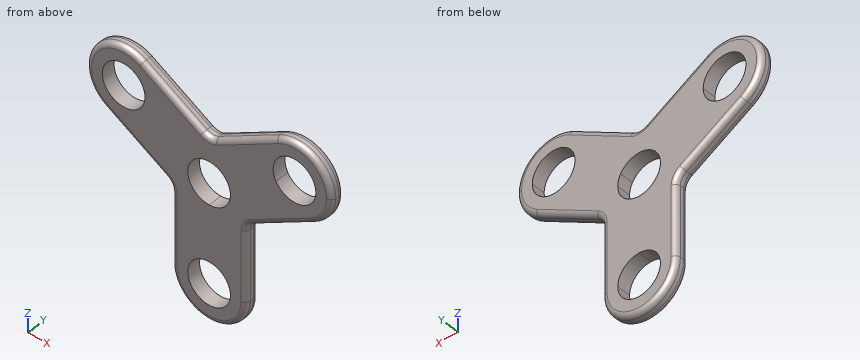
from build123d import *

# Parameters (mm, degrees)
F1_DEPTH = 6.9977
F2_R     = 2.54


with BuildPart() as f1:
    # F0 (on Front) → F1 (new body)
    with BuildSketch(Plane.XZ):
        with BuildLine():
            ThreePointArc((16.4977839421, 15.875), (18.4008869908, 11.2805028092), (19.05, 6.35))
            ThreePointArc((19.05, 6.35), (13.4703841816, -7.1203841816), (0, -12.7))
            Line((0, -12.7), (0, -25.4))
            ThreePointArc((0, -25.4), (13.4703841816, -30.9796158184), (19.05, -44.45))
            Line((19.05, -44.45), (19.05, -8.3146968374))
            ThreePointArc((19.05, -8.3146968374), (19.900738686, -5.1396968374), (22.225, -2.8154355234))
            Line((22.225, -2.8154355234), (53.5190905122, 15.2522160579))
            ThreePointArc((53.5190905122, 15.2522160579), (39.063587703, 13.3491130092), (27.4963065702, 22.225))
            Line((27.4963065702, 22.225), (16.4977839421, 15.875))
        make_face()
        with BuildLine():
            ThreePointArc((-16.4977839421, 15.875), (0, 25.4), (16.4977839421, 15.875))
            Line((16.4977839421, 15.875), (27.4963065702, 22.225))
            ThreePointArc((27.4963065702, 22.225), (25.5932035214, 36.6805028092), (34.4690905122, 48.2477839421))
            Line((34.4690905122, 48.2477839421), (3.175, 30.1801323608))
            ThreePointArc((3.175, 30.1801323608), (0, 29.3293936748), (-3.175, 30.1801323608))
            Line((-3.175, 30.1801323608), (-34.4690905122, 48.2477839421))
            ThreePointArc((-34.4690905122, 48.2477839421), (-27.4963065702, 41.275), (-24.9440905122, 31.75))
            ThreePointArc((-24.9440905122, 31.75), (-25.5932035214, 26.8194971908), (-27.4963065702, 22.225))
            Line((-27.4963065702, 22.225), (-16.4977839421, 15.875))
        make_face()
        with BuildLine():
            Line((0, -25.4), (0, -12.7))
            ThreePointArc((0, -12.7), (-16.4977839421, -3.175), (-16.4977839421, 15.875))
            Line((-16.4977839421, 15.875), (-27.4963065702, 22.225))
            ThreePointArc((-27.4963065702, 22.225), (-39.063587703, 13.3491130092), (-53.5190905122, 15.2522160579))
            Line((-53.5190905122, 15.2522160579), (-22.225, -2.8154355234))
            ThreePointArc((-22.225, -2.8154355234), (-19.900738686, -5.1396968374), (-19.05, -8.3146968374))
            Line((-19.05, -8.3146968374), (-19.05, -44.45))
            ThreePointArc((-19.05, -44.45), (-13.4703841816, -30.9796158184), (0, -25.4))
        make_face()
        with BuildLine():
            ThreePointArc((34.4690905122, 48.2477839421), (25.5932035214, 36.6805028092), (27.4963065702, 22.225))
            ThreePointArc((27.4963065702, 22.225), (39.063587703, 13.3491130092), (53.5190905122, 15.2522160579))
            ThreePointArc((53.5190905122, 15.2522160579), (60.4918744543, 22.225), (63.0440905122, 31.75))
            ThreePointArc((63.0440905122, 31.75), (53.5190905122, 48.2477839421), (34.4690905122, 48.2477839421))
        make_face()
        with BuildLine():
            ThreePointArc((54.9940939122, 31.75), (46.8411008884, 21.1248126267), (34.4678081261, 26.2499983))
            ThreePointArc((34.4678081261, 26.2499983), (41.1470801361, 42.3751873733), (54.9940939122, 31.75))
        make_face(mode=Mode.SUBTRACT)
        with BuildLine():
            ThreePointArc((19.05, -44.45), (13.4703841816, -30.9796158184), (0, -25.4))
            ThreePointArc((0, -25.4), (-13.4703841816, -30.9796158184), (-19.05, -44.45))
            ThreePointArc((-19.05, -44.45), (0, -63.5), (19.05, -44.45))
        make_face()
        with BuildLine():
            ThreePointArc((11.0000034, -44.45), (-7.7781769972, -52.2281769972), (0, -33.4499966))
            ThreePointArc((0, -33.4499966), (7.7781769972, -36.6718230028), (11.0000034, -44.45))
        make_face(mode=Mode.SUBTRACT)
        with BuildLine():
            ThreePointArc((-53.5190905122, 15.2522160579), (-39.063587703, 13.3491130092), (-27.4963065702, 22.225))
            ThreePointArc((-27.4963065702, 22.225), (-25.5932035214, 26.8194971908), (-24.9440905122, 31.75))
            ThreePointArc((-24.9440905122, 31.75), (-27.4963065702, 41.275), (-34.4690905122, 48.2477839421))
            ThreePointArc((-34.4690905122, 48.2477839421), (-60.4918744543, 41.275), (-53.5190905122, 15.2522160579))
        make_face()
        with BuildLine():
            ThreePointArc((-32.9940871122, 31.75), (-33.3689031389, 28.9029896239), (-34.4678081261, 26.2499983))
            ThreePointArc((-34.4678081261, 26.2499983), (-54.6192778856, 34.5970103761), (-32.9940871122, 31.75))
        make_face(mode=Mode.SUBTRACT)
        with BuildLine():
            ThreePointArc((-16.4977839421, 15.875), (-16.4977839421, -3.175), (0, -12.7))
            Line((0, -12.7), (0, -4.6500034))
            ThreePointArc((0, -4.6500034), (-9.5262823861, 0.8499983), (-9.5262823861, 11.8500017))
            Line((-9.5262823861, 11.8500017), (-16.4977839421, 15.875))
        make_face()
        with BuildLine():
            ThreePointArc((0, -12.7), (13.4703841816, -7.1203841816), (19.05, 6.35))
            ThreePointArc((19.05, 6.35), (18.4008869908, 11.2805028092), (16.4977839421, 15.875))
            Line((16.4977839421, 15.875), (9.5262823861, 11.8500017))
            ThreePointArc((9.5262823861, 11.8500017), (10.6251873733, 9.1970103761), (11.0000034, 6.35))
            ThreePointArc((11.0000034, 6.35), (7.7781769972, -1.4281769972), (0, -4.6500034))
            Line((0, -4.6500034), (0, -12.7))
        make_face()
        with BuildLine():
            Line((9.5262823861, 11.8500017), (16.4977839421, 15.875))
            ThreePointArc((16.4977839421, 15.875), (0, 25.4), (-16.4977839421, 15.875))
            Line((-16.4977839421, 15.875), (-9.5262823861, 11.8500017))
            ThreePointArc((-9.5262823861, 11.8500017), (0, 17.3500034), (9.5262823861, 11.8500017))
        make_face()
    extrude(amount=F1_DEPTH)

    # F2
    f2_edges = [f1.edges().sort_by_distance(p)[0] for p in [
        (0, -6.9977, -63.5),
        (0, 0, -63.5),
    ]]
    fillet(f2_edges, radius=F2_R)


solid = f1.part
Source: CAD feature listing. Evaluate the final solid. Frame: model axes, mm. Coordinates: 2 decimals unless noted, no trailing zeros. Loops run counter-clockwise (first coordinate to the right, second up) from the corner with the lowest first, then second, coordinate; pieces in that order, holes last. Notation, with made-up numbers: (-30, 23) - (-21, 23) arc R23 ccw to (-21, 53) - close; hole circle Ø5 at (-19.75, 26). An arc over 180 degrees is marked (long way). Return JSON: item names as keys, results as strings.
Q1. Section A-A, the plane z = -21.5. Return loops of the section in (x, y).
Results:
{"outline": "(-19.05, -4.46) arc R2.54 ccw to (-16.51, -7) - (16.51, -7) arc R2.54 ccw to (19.05, -4.46) - (19.05, -2.54) arc R2.54 ccw to (16.51, 0) - (-16.51, 0) arc R2.54 ccw to (-19.05, -2.54) - close"}
Q2. Contact query for flat-ended pins moving along their axis: P1, Ø1, axis at y = -4, z = -7.5, coming from the +X side; P2, Ø1.5, axis at x = 32, y = -6, coming from the -Z side; P3, Ø4, axis at y = -5, z = -21.5, coming from the -X side; P4, Ø17.5, axis at x = 43.99, z = 31.75, coming from the +Y side. Output: stop coordinate, or through.
Results:
{"P1": "x = 19.19", "P2": "z = 2.76", "P3": "x = -19.05", "P4": "through"}
Q3. Material intervals for line 1 along X through (y, z) = (-3.25, -44.45); line 2 along X through (y, z) = (-3, 31.75); line 3 along Z through (x, y) = (10, -4.25), sorted ascending.
Results:
{"line 1": "-19.05 to -11, 11 to 19.05", "line 2": "-63.04 to -54.99, -32.99 to -5.89, 5.89 to 32.99, 54.99 to 63.04", "line 3": "-60.66 to -49.03, -39.87 to 1.77, 10.93 to 34.12"}
Q4. Section C-C, the plane x = 7. Give the number of separate pieces and of enclosed holes in the cut face, plus the area to 3 significant figures.
Results:
{"separate pieces": "3", "enclosed holes": "0", "area": "418 mm2"}
